Geometry check sheet. Reference: the model listing, model coordinates, mm. Round coordinates to 2 decimals unless told otherwise and drop trailing zeros. Loops run counter-clockwise (first coordinate to the right, second up) from the corner with the lowest first, then second, coordinate; pieces in that order, holes last.
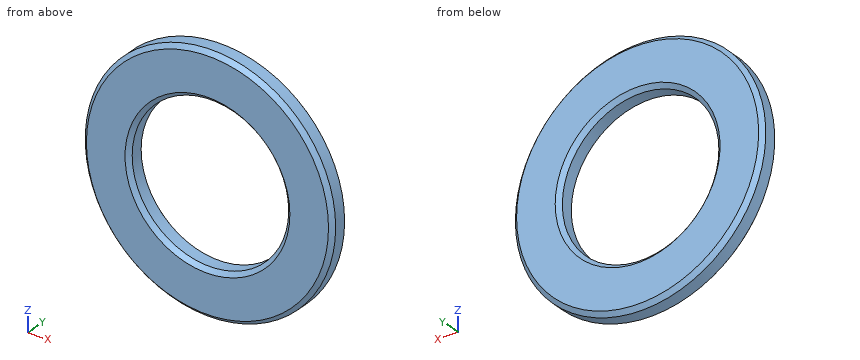
```python
from build123d import *

# Parameters (mm, degrees)
F0_R     = 38.1
F0_R_2   = 23.8125
F1_DEPTH = 3.175
F2_SIZE  = 1.27


with BuildPart() as f1:
    # F0 (on Front) → F1 (new body, symmetric)
    with BuildSketch(Plane.XZ):
        Circle(F0_R)
        Circle(F0_R_2, mode=Mode.SUBTRACT)
    extrude(amount=F1_DEPTH, both=True)

    # F2
    f2_edges = [f1.edges().sort_by_distance(p)[0] for p in [
        (-38.1, 3.175, 0),
        (38.1, 0, 0),
        (-38.1, -3.175, 0),
        (-23.8125, -3.175, 0),
        (23.8125, 0, 0),
        (-23.8125, 3.175, 0),
    ]]
    chamfer(f2_edges, length=F2_SIZE)


solid = f1.part
```
1) Gauge pin test, flat ends, axial feed: pin 1 (2 mm diameter, centred on y = -1, z = -7, fed in from +X); pin 2 (1 mm diameter, centred on y = 2, z = -30, fed in from -X). Record the tip position at first contact, or that the pin passes through.
Report:
pin 1: stops at x = 37.62
pin 2: stops at x = -24.1
2) Sectioned sample at A-A, the plane z = 0. Record the cut outline in (x, y) (1 decimal).
Report:
outline: (-38.1, -1.9) - (-36.8, -3.2) - (-25.1, -3.2) - (-23.8, -1.9) - (-23.8, 1.9) - (-25.1, 3.2) - (-36.8, 3.2) - (-38.1, 1.9) - close; (23.8, -1.9) - (25.1, -3.2) - (36.8, -3.2) - (38.1, -1.9) - (38.1, 1.9) - (36.8, 3.2) - (25.1, 3.2) - (23.8, 1.9) - close
3) Sectioned sample at B-B, the plane x = 0. Record the cut outline in (y, z) (1 decimal).
Report:
outline: (-3.2, -36.8) - (-1.9, -38.1) - (1.9, -38.1) - (3.2, -36.8) - (3.2, -25.1) - (1.9, -23.8) - (-1.9, -23.8) - (-3.2, -25.1) - close; (-3.2, 25.1) - (-1.9, 23.8) - (1.9, 23.8) - (3.2, 25.1) - (3.2, 36.8) - (1.9, 38.1) - (-1.9, 38.1) - (-3.2, 36.8) - close
4) Scan lines: line 1 along Z through (x, y) = (11, -2.5); line 2 along Z through (x, y) = (0, -0.65); line 3 along X through (y, z) = (3, -1.5). Record each from-to range of solid material in increasing order.
Report:
line 1: z = -35.86 to -21.79, 21.79 to 35.86
line 2: z = -38.1 to -23.81, 23.81 to 38.1
line 3: x = -36.97 to -24.86, 24.86 to 36.97
5) Sectioned sample at C-C, the plane y = 0. Record the cut outline in (x, z) (1 decimal), then the cut area to 3 significant figures.
Report:
outline: circle Ø76.2 at (0, 0); hole circle Ø47.6 at (0, 0)
area: 2,780 mm2
